from build123d import *

# Parameters (mm, degrees)
ESBO_O1_R                                      = 4.7625
RESSALTO_EXTRUS_O1_DEPTH                       = 78
FURO_ROSCADO_DE_M3X0_52_D                      = 2.5
FURO_ROSCADO_DE_M3X0_52_DEPTH                  = 8.5
FURO_ROSCADO_DE_M3X0_52_TIP                    = 0.751075774
FILETE1_R                                      = 0.5
BROCA_DE_ROSQUEAR_PARA_TARRAXA_DE_M3X0_5_D     = 2.5
BROCA_DE_ROSQUEAR_PARA_TARRAXA_DE_M3X0_5_DEPTH = 5
BROCA_DE_ROSQUEAR_PARA_TARRAXA_DE_M3X0_5_TIP   = 0.751075774
FILETE2_R                                      = 0.5


with BuildPart() as part:
    # Esboço1 → Ressalto-extrusão1 (new body)
    with BuildSketch(Plane.XY):
        with Locations((240.708388302, 2.596082859)):
            Circle(ESBO_O1_R)
    extrude(amount=RESSALTO_EXTRUS_O1_DEPTH)

    # Furo roscado de M3x0.52
    with Locations(Plane(origin=(0, 0, 0), x_dir=(-1, 0, 0), z_dir=(0, 0, -1))):
        with Locations((-240.708388302, 2.596082859)):
            Hole(FURO_ROSCADO_DE_M3X0_52_D / 2, depth=FURO_ROSCADO_DE_M3X0_52_DEPTH)
            with Locations((0, 0, -(FURO_ROSCADO_DE_M3X0_52_DEPTH + FURO_ROSCADO_DE_M3X0_52_TIP / 2))):  # 118° drill point
                Cone(0, FURO_ROSCADO_DE_M3X0_52_D / 2, FURO_ROSCADO_DE_M3X0_52_TIP, mode=Mode.SUBTRACT)

    # Filete1
    filete1_edges = [part.edges().sort_by_distance(p)[0] for p in [
        (235.945888302, 2.596082859, 0),
    ]]
    fillet(filete1_edges, radius=FILETE1_R)

    # Broca de rosquear para tarraxa de M3x0.51
    with Locations(Plane.XY.offset(78)):
        with Locations((240.708388302, 2.596082859)):
            Hole(BROCA_DE_ROSQUEAR_PARA_TARRAXA_DE_M3X0_5_D / 2, depth=BROCA_DE_ROSQUEAR_PARA_TARRAXA_DE_M3X0_5_DEPTH)
            with Locations((0, 0, -(BROCA_DE_ROSQUEAR_PARA_TARRAXA_DE_M3X0_5_DEPTH + BROCA_DE_ROSQUEAR_PARA_TARRAXA_DE_M3X0_5_TIP / 2))):  # 118° drill point
                Cone(0, BROCA_DE_ROSQUEAR_PARA_TARRAXA_DE_M3X0_5_D / 2, BROCA_DE_ROSQUEAR_PARA_TARRAXA_DE_M3X0_5_TIP, mode=Mode.SUBTRACT)

    # Filete2
    filete2_edges = [part.edges().sort_by_distance(p)[0] for p in [
        (235.945888302, 2.596082859, 78),
    ]]
    fillet(filete2_edges, radius=FILETE2_R)


solid = part.part
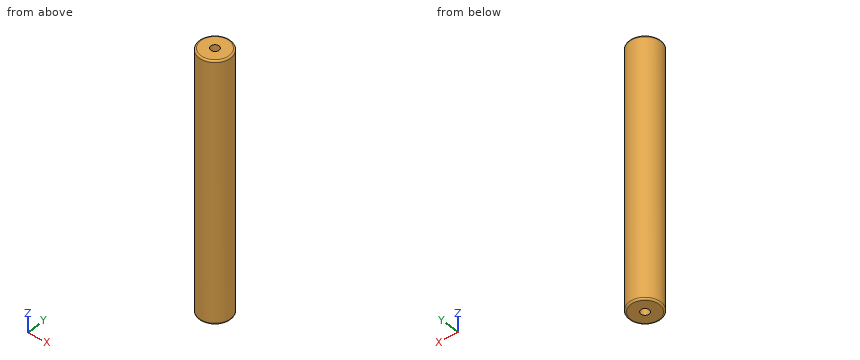
Geometry: final body of the model. Coordinates: model frame, mm. Coordinates: 2 decimals unless noted, no trailing zeros. Order: outer loops, then holes, each group sorted by start corner. A loop starts at its lowest first (then second) coordinate and runs counter-clockwise, first axis right, second up.
1) Section B-B (z = 60). Return loops of the section in (x, y) (1 decimal), then the cut area to 3 significant figures.
Result sheet:
outline: circle Ø9.5 at (240.7, 2.6)
area: 71.3 mm2
2) First-contact query: P1, Ø1, axis at x = 242, z = 15, coming from the +Y side; P2, Ø2, axis at x = 239, z = 40.5, coming from the -Y side; P3, Ø2, axis at x = 240.71, y = 2.6, coming from the +Z side. Flat tips, straight axial feed; report the tip coordinate or a pass-through.
Result sheet:
P1: stops at y = 7.29
P2: stops at y = -2.11
P3: stops at z = 72.85
3) Ray query, probe 1 along Y at (x, z) = (241, 63.5); probe 2 along Z at (x, y) = (245, 1.75); probe 3 along X at (y, z) = (5.5, 11). Return the intervals inside material, ascending.
Result sheet:
probe 1: y = -2.16 to 7.35
probe 2: z = 0.01 to 77.99
probe 3: x = 236.93 to 244.48
